The model under review builds one solid part; all positions refer to its coordinate system, in mm. A direction names the side the tool comes from. Coordinates: 2 decimals unless noted, no trailing zeros. Order: outer loops, then holes, each group sorted by start corner. A loop starts at its lowest first (then second) coordinate and runs counter-clockwise, first axis right, second up. Notation, with made-up numbers: M 29,19.5 L 85,19.5 A18 ccw 85,48.5 Z; hole C 71,-19.75 d10. An arc over 180 degrees is marked long. Answer as CSV lines item,"result". Start each with the question number.
Q1. Wall thickness on L1, parallel to Z at x = 5.25, y = 0; L2, parallel to Y at x = 8, z = 4.75; L3, parallel to Y at x = 7, z = 1.75: over which ranges is each line inside the solid? List them lowest first. Write a range as [from, to].
Q2. Consider section A-A on z = 6. Write out the cut boundary in (x, y), and give its area (3 significant figures).
Q3. The part is to be moulded in two halves that separate along X. For faces 5 (the face through (0, 0, 0)), 6 (the face through (0, -3, 6)), 7 (the face through (9, 5, 2)), say which applies: +X half, -X half, draft (parallel to the pull), parting line (faces both ways), or undercut.
Q4. Consider section B-B on x = 0. Write out the cut boundary in (y, z), and give its area (3 significant figures).
Q5. Consider section C-C on y = 0. Write out the cut boundary in (x, z), and give its area (3 significant figures).
Q6. Consider section D-D on z = 1.5. Write out the cut boundary in (x, y), and give its area (3 significant figures).
Q7. For P1, Ø4, axis at x = 6, y = -5, coming from the +Z side; P2, Ø1.5, axis at x = 9.5, z = 3, coming from the +Y side; P3, Ø0.6, axis at x = -9, z = 2.5, coming from the +Y side, all flat-tipped, find the tip position at first contact; note any pin that passes through.
Q8. Machinability: for faces 1 (the face through (-9, 1.5, 3)), 2 (the face through (0, -5, 6)), 3 (the face through (0, 3.5, 6)), 4 (the face through (6.5, 0, 2.5)), which of the approach directions +Z, -Z, +X, -X, +Y, -Y give a long, thin tool a straight path to every point of the face, cutting with its end or side? Answer none if there is none.
from build123d import *

# Parameters (mm, degrees)
BOSS_EXTRUDE2_DEPTH = 5
CUT_EXTRUDE1_DEPTH  = 5
SKETCH3_R           = 0.5
BOSS_EXTRUDE3_DEPTH = 3
BOSS_EXTRUDE4_DEPTH = 2
SKETCH5_W           = 5
SKETCH5_H           = 1
CUT_EXTRUDE2_DEPTH  = 2


with BuildPart() as part:
    # Sketch1 → Boss-Extrude2 (new body)
    with BuildSketch(Plane.XY):
        with BuildLine():
            ThreePointArc((-6.955420634, 8.36), (-9.215164105, 4.44856897), (-10, 0))
            Line((-10, 0), (10, 0))
            ThreePointArc((10, 0), (9.215164105, 4.44856897), (6.955420634, 8.36))
            Line((6.955420634, 8.36), (-6.955420634, 8.36))
        make_face()
        with BuildLine():
            Line((10, 0), (-10, 0))
            ThreePointArc((-10, 0), (-9.215164105, -4.44856897), (-6.955420634, -8.36))
            Line((-6.955420634, -8.36), (6.955420634, -8.36))
            ThreePointArc((6.955420634, -8.36), (9.215164105, -4.44856897), (10, 0))
        make_face()
    extrude(amount=BOSS_EXTRUDE2_DEPTH)

    # Sketch2 → Cut-Extrude1 (cut)
    with BuildSketch(Plane.XY.offset(5)):
        with BuildLine():
            Line((-8, 1.5), (-9.91317157, 1.5))
            Line((-9.91317157, 1.5), (-10.317130361, 1.5))
            ThreePointArc((-10.317130361, 1.5), (-10.425602087, 0), (-10.317130361, -1.5))
            Line((-10.317130361, -1.5), (-9.91317157, -1.5))
            Line((-9.91317157, -1.5), (-8, -1.5))
            ThreePointArc((-8, -1.5), (-6.5, 0), (-8, 1.5))
        make_face()
        with BuildLine():
            Line((8, -1.5), (9.91317157, -1.5))
            Line((9.91317157, -1.5), (10.317130361, -1.5))
            ThreePointArc((10.317130361, -1.5), (10.425602087, 0), (10.317130361, 1.5))
            Line((10.317130361, 1.5), (9.91317157, 1.5))
            Line((9.91317157, 1.5), (8, 1.5))
            ThreePointArc((8, 1.5), (6.5, 0), (8, -1.5))
        make_face()
    extrude(amount=-CUT_EXTRUDE1_DEPTH, mode=Mode.SUBTRACT)

    # Sketch3 → Boss-Extrude3 (add)
    with BuildSketch(Plane.XY.offset(5)):
        Circle(SKETCH3_R)
    extrude(amount=BOSS_EXTRUDE3_DEPTH)

    # Sketch4 → Boss-Extrude4 (add)
    with BuildSketch(Plane.XY.offset(5)):
        with BuildLine():
            Line((-3.570714214, 3.5), (3.570714214, 3.5))
            ThreePointArc((3.570714214, 3.5), (0, -5), (-3.570714214, 3.5))
        make_face()
    extrude(amount=BOSS_EXTRUDE4_DEPTH)

    # Sketch5 → Cut-Extrude2 (cut)
    with BuildSketch(Plane.XY.offset(7)):
        with Locations((0, -2.5)):
            Rectangle(SKETCH5_W, SKETCH5_H)
    extrude(amount=-CUT_EXTRUDE2_DEPTH, mode=Mode.SUBTRACT)


solid = part.part
Evaluation:
1,L1,"z = [0, 5]"
1,L2,"y = [-6.93, -1.5], [1.5, 6.93]"
1,L3,"y = [-8.31, -1.12], [1.12, 8.31]"
2,outline,"M -3.57,3.5 A5 ccw long 3.57,3.5 Z; hole M -2.5,-3 L 2.5,-3 L 2.5,-2 L -2.5,-2 Z"
2,area,"66.2 mm²"
3,face 5,"draft"
3,face 6,"undercut"
3,face 7,"+X half"
4,outline,"M -8.36,0 L 8.36,0 L 8.36,5 L 3.5,5 L 3.5,7 L 0.5,7 L 0.5,8 L -0.5,8 L -0.5,7 L -2,7 L -2,5 L -3,5 L -3,7 L -5,7 L -5,5 L -8.36,5 Z"
4,area,"99.6 mm²"
5,outline,"M -6.5,0 L 6.5,0 L 6.5,5 L 5,5 L 5,7 L 0.5,7 L 0.5,8 L -0.5,8 L -0.5,7 L -5,7 L -5,5 L -6.5,5 Z"
5,area,"86.0 mm²"
6,outline,"M -9.91,-1.5 A13 ccw -6.96,-8.36 L 6.96,-8.36 A13 ccw 9.91,-1.5 L 8,-1.5 A1.5 cw 8,1.5 L 9.91,1.5 A13 ccw 6.96,8.36 L -6.96,8.36 A13 ccw -9.91,1.5 L -8,1.5 A1.5 cw -8,-1.5 Z"
6,area,"283 mm²"
7,P1,"stops at z = 5"
7,P2,"stops at y = 5.56"
7,P3,"stops at y = 5.67"
8,face 1,"+Z, -Z, -X"
8,face 2,"+Z"
8,face 3,"+Z, +X, -X, +Y"
8,face 4,"+Z, -Z, +X"
